Here's how the part is built. I have some questions about the finished solid (model axes, mm). Face numbers are marked on the shaded views. A direction names the side the tool comes from. Round coordinates to 2 decimals unless told otherwise and drop trailing zeros. Write each loop counter-clockwise with the first axis right and the second up, starting at its lowest first coordinate (ties: lowest second). Pieces come first, ordered by that corner, then holes. Notation, with made-up numbers: (30, 30.25) -> (77, 30.25) arc R14 ccw to (77, 53.25) -> close; hole circle Ø6 at (34, -33.5). An arc over 180 degrees is marked (long way). Answer as CSV lines item,"result".
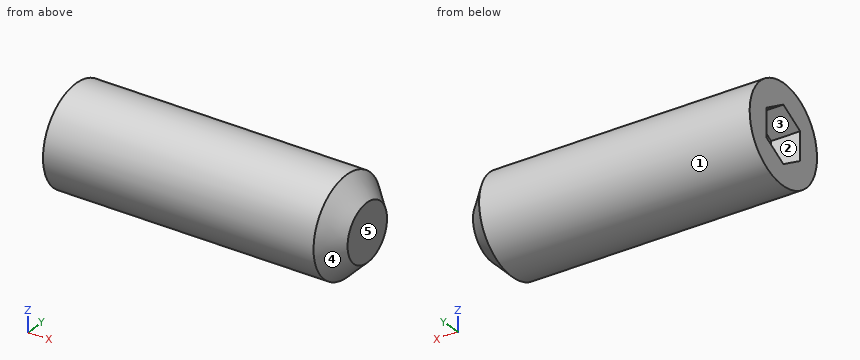
from build123d import *

# Parameters (mm, degrees)
CUT_EXTRUDE1_DEPTH = 3


with BuildPart() as part:
    # Sketch1 → Revolve1 (revolve)
    with BuildSketch(Plane.XY, mode=Mode.PRIVATE) as revolve1_sk:
        Polygon((30, 2.928932188), (30, 0), (0, 0), (0, 5), (27.928932188, 5), align=None)
    revolve(revolve1_sk.sketch.rotate(Axis((0, 0, 0), (1, 0, 0)), 90), axis=Axis((0, 0, 0), (1, 0, 0)))

    # Sketch2 → Cut-Extrude1 (cut)
    with BuildSketch(Plane.ZY):
        Polygon((-1.443375673, 2.5), (-2.886751346, 0), (-1.443375673, -2.5), (1.443375673, -2.5), (2.886751346, 0), (1.443375673, 2.5), align=None)
    extrude(amount=-CUT_EXTRUDE1_DEPTH, mode=Mode.SUBTRACT)


solid = part.part
Item 1: Will these pins go through, and if not, where does the flat tip stop? pin 1 (3 mm diameter, centred on x = 1.5, z = 0.5, fed in from -Y); pin 2 (1 mm diameter, centred on x = 13.5, y = 2.5, fed in from +Z); pin 3 (1.5 mm diameter, centred on x = 8.5, y = -2.5, fed in from -Z); pin 4 (2.5 mm diameter, centred on y = 0.5, z = -1, fed in from -X).
Results found:
pin 1,"stops at y = -5"
pin 2,"stops at z = 4.58"
pin 3,"stops at z = -4.68"
pin 4,"stops at x = 3"
Item 2: If we mould it in two halves opening along Y, with no side actions, what happens to the marked faces 3, 4 and 5? For each: pulls with the +Y half, pulls with the -Y half, needs draft (parallel to the pull), parting line crosses it, or undercut.
Results found:
face 3,"undercut"
face 4,"parting line crosses it"
face 5,"needs draft"
Item 3: For the marked faces 1 and 2, which set-ups out of +Z, -Z, +X, -X, +Y, -Y let a thin tool reach every point of the face, with its end or its side?
Results found:
face 1,"+X, -X"
face 2,"-X"
Item 4: I need wall thicknesses on L1, parallel to X at y = 2, z = 0.25; L2, parallel to Z at x = 2.75, y = 0.5; L3, parallel to Y at x = 7.5, z = 4.5. Which ranges of each line are inside material? Lowest first, please.
Results found:
L1,"x = 3 to 30"
L2,"z = -4.97 to -2.6, 2.6 to 4.97"
L3,"y = -2.18 to 2.18"
Item 5: Suppose I cut it at B-B, the plane x = 4.5. List the corners of the cut face in (y, z) for me, then the cut area to 3 significant figures.
Results found:
outline,"circle Ø10 at (0, 0)"
area,"78.5 mm²"
Item 6: Suppose I cut it at A-A, the plane z = 0. List the corners of the cut face in (x, y) for me.
Results found:
outline,"(0, -5) -> (27.93, -5) -> (30, -2.93) -> (30, 2.93) -> (27.93, 5) -> (0, 5) -> (0, 2.5) -> (3, 2.5) -> (3, -2.5) -> (0, -2.5) -> close"
